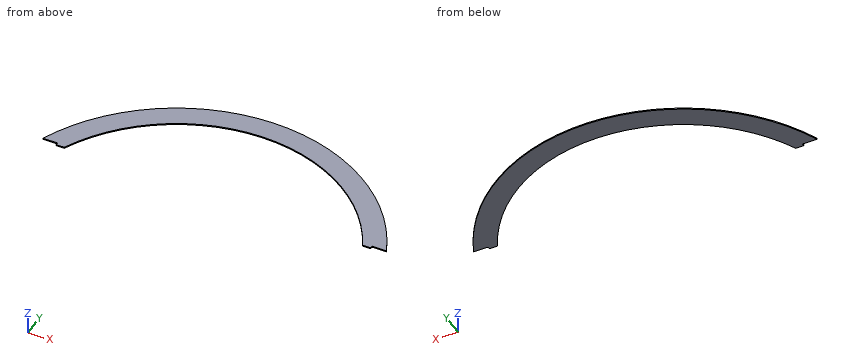
from build123d import *

# Parameters (mm, degrees)
SKETCH1_R          = 950
SKETCH1_R_2        = 840
BASE_FLANGE1_DEPTH = 6
SKETCH6_W          = 2732.981099596
SKETCH6_H          = 1353.854573776
CUT_EXTRUDE1_DEPTH = 10
SKETCH8_W          = 79.396529378
SKETCH8_H          = 13
CUT_EXTRUDE2_DEPTH = 10


# Sheet-metal steps are written as plain solids
with BuildPart() as part:
    # Sketch1 → Base-Flange1 (new body)
    with BuildSketch(Plane.XY):
        Circle(SKETCH1_R)
        Circle(SKETCH1_R_2, mode=Mode.SUBTRACT)
    extrude(amount=-BASE_FLANGE1_DEPTH)

    # Sketch6 → Cut-Extrude1 (cut)
    with BuildSketch(Plane.XY):
        with Locations((-160.657409421, -313.927286888)):
            Rectangle(SKETCH6_W, SKETCH6_H)
    extrude(amount=-CUT_EXTRUDE1_DEPTH, mode=Mode.SUBTRACT)

    # Sketch8 → Cut-Extrude2 (cut)
    with BuildSketch(Plane.XY):
        with Locations((-838.214601147, 369.5)):
            Rectangle(SKETCH8_W, SKETCH8_H)
    cut_extrude2 = extrude(amount=-CUT_EXTRUDE2_DEPTH, mode=Mode.SUBTRACT)

    # Mirror1: Cut-Extrude2 across plane
    add(cut_extrude2.mirror(Plane(origin=(0, 0, 0), x_dir=(0, 0, 1), z_dir=(1, 0, 0))), mode=Mode.SUBTRACT)


solid = part.part
Here's how the part is built. I have some questions about the finished solid (model axes, mm). Coordinates: 2 decimals unless noted, no trailing zeros. Loops run counter-clockwise (first coordinate to the right, second up) from the corner with the lowest first, then second, coordinate; pieces in that order, holes last.
1. Imagine slicing it at B-B, the plane z = -1.65. Please give me the cut outline in (x, y), and give its area (3 significant figures).
2. I need wall thicknesses on L1, parallel to X at y = 606, z = -4.65; L2, parallel to X at y = 522, z = -4.35; L3, parallel to Y at x = 531, z = -2.7. Which ranges of each line are inside material? Lowest first, please.
3. For P1, Ø1.8, axis at x = 818, z = -1.5, coming from the -Y side; P2, Ø1.8, axis at y = 368.5, z = -1.5, coming from the +X side; P3, Ø3, axis at y = 701.5, z = -4.5, coming from the +X side, each with a flat end and sliding along its axis, tell me the tip position at first contact or that it passes through.
4. Imagine slicing it at D-D, the plane y = 537. Please give me the cut outline in (x, z).
5. Imagine slicing it at C-C, the plane x = -343. Please give me the cut outline in (y, z), and give its area (3 significant figures).
6. Imagine slicing it at A-A, the plane y = 751. Please give me the cut outline in (x, z), and give its area (3 significant figures).
Taken from the geometry:
1. outline: (-872.42, 376) - (-798.52, 376) - (-798.52, 363) - (-757.52, 363) arc R840 cw to (757.52, 363) - (798.52, 363) - (798.52, 376) - (872.42, 376) arc R950 ccw to start
1. area: 225,000 mm2
2. L1: x = -731.62 to -581.69, 581.69 to 731.62
2. L2: x = -793.74 to -658.12, 658.12 to 793.74
2. L3: y = 650.88 to 787.74
3. P1: stops at y = 376
3. P2: stops at x = 798.52
3. P3: stops at x = 642.26
4. outline: (-783.67, -6) - (-645.93, -6) - (-645.93, 0) - (-783.67, 0) - close; (645.93, -6) - (783.67, -6) - (783.67, 0) - (645.93, 0) - close
5. outline: (766.78, -6) - (885.92, -6) - (885.92, 0) - (766.78, 0) - close
5. area: 715 mm2
6. outline: (-581.81, -6) - (-376.3, -6) - (-376.3, 0) - (-581.81, 0) - close; (376.3, -6) - (581.81, -6) - (581.81, 0) - (376.3, 0) - close
6. area: 2,470 mm2
